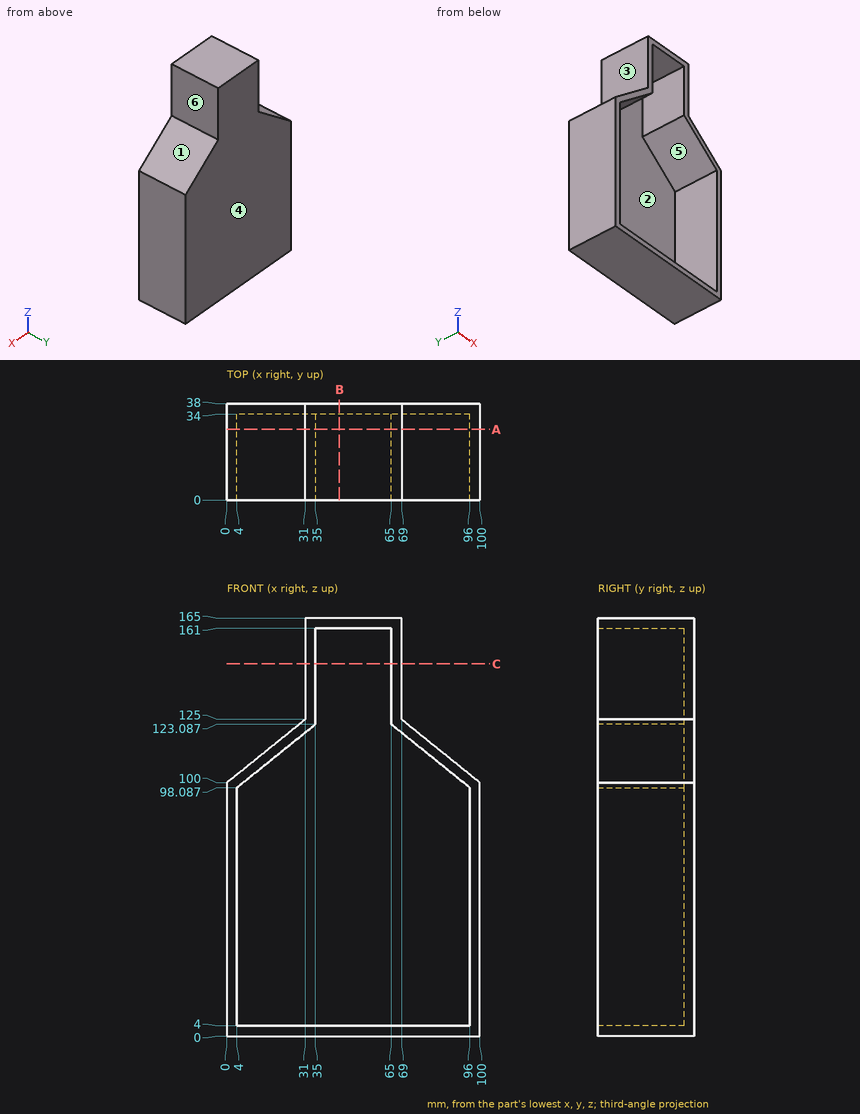
Input: dimensioned drawing with shaded views. Units: mm. Origin: part minimum x, y, z. A direction names the side the tool comes from. Round coordinates to 2 decimals unless told otherwise and drop trailing zeros. Loops run counter-clockwise (first coordinate to the right, second up) from the corner with the lowest first, then second, coordinate; pieces in that order, holes last. Notation, with made-up numbers: (63.25, -14.75) -> (77.25, -14.75) arc R10 ccw to (77.25, -5.75) -> close; hole circle Ø9 at (42, 67.5). An arc over 180 degrees is marked (long way). Use one line per item in the form item = value. Start each with the question number.
1) First-contact query: P1, Ø10, axis at y = 22.5, z = 146, coming from the +X side; P2, Ø5, axis at x = 38, z = 58, coming from the -Y side; P3, Ø1.5, axis at x = 19, y = 13, coming from the +Z side. Flat tips, straight axial feed; report the tip coordinate or a pass-through.
2) Access query for the marked faces 1, 2 and 3. Directions: +Z, -Z, +X, -X, +Y, -Y. A direction counts if a zero-diameter tool reaches every point of the face in a straight line with its end or side. Return the directions, or none.
3) Draft query along X for the marked faces 4, 5 and 6. Return one class per face: released by +X, released by -X, zero draft, split by the parting line, or undercut.
4) Section B-B on x = 44.5. Output: boundary loops of the cut face in (y, z), then the cut area to 3 significant figures.
5) Line query: L1, parallel to Z at x = 37, y = 31; L2, parallel to X at y = 23, z = 97; L3, parallel to X at y = 13.5, z = 155.5. Output: solid intervals per line, ascending.
6) Section A-A on y = 28. Output: boundary loops of the cut face in (x, z).
7) Section C-C on z = 147. Output: boundary loops of the cut face in (x, y).
Response:
q1.P1 = 69
q1.P2 = 34
q1.P3 = 115.93
q2.face_1 = +Z, +X, +Y, -Y
q2.face_2 = -Y
q2.face_3 = +Z, -X, +Y, -Y
q3.face_4 = zero draft
q3.face_5 = undercut
q3.face_6 = released by +X
q4.outline = (0, 0) -> (38, 0) -> (38, 165) -> (0, 165) -> (0, 161) -> (34, 161) -> (34, 4) -> (0, 4) -> close
q4.area = 932 mm^2
q5.L1 = 0 to 4, 161 to 165
q5.L2 = 0 to 4, 96 to 100
q5.L3 = 31 to 35, 65 to 69
q6.outline = (0, 0) -> (100, 0) -> (100, 100) -> (69, 125) -> (69, 165) -> (31, 165) -> (31, 125) -> (0, 100) -> close; hole (4, 4) -> (96, 4) -> (96, 98.09) -> (65, 123.09) -> (65, 161) -> (35, 161) -> (35, 123.09) -> (4, 98.09) -> close
q7.outline = (31, 0) -> (35, 0) -> (35, 34) -> (65, 34) -> (65, 0) -> (69, 0) -> (69, 38) -> (31, 38) -> close
